from build123d import *

# Parameters (mm, degrees)
F0_W      = 130.6354291737
F0_H      = 70.8588063717
F1_DEPTH  = 25.4
F2_W      = 21.0115239024
F2_H      = 16.2068661302
F3_DEPTH  = 139.7
F4_W      = 130.6354291737
F4_H      = 35.4294031858
F5_DEPTH  = 27.94
F7_DEPTH  = 157.48
F8_W      = 13.1810824387
F8_H      = 8.3256293517
F8_W_2    = 15.867670998
F9_DEPTH  = 147.32
F10_W     = 5.3731799126
F10_H     = 22.795913741
F11_DEPTH = 15.24
F13_DEPTH = 25.4
F14_W     = 5.5410936475
F14_H     = 23.0333786458
F15_DEPTH = 15.24
F17_DEPTH = 25.4
F19_DEPTH = 45.72


with BuildPart() as f1:
    # F0 (on Top) → F1 (new body)
    with BuildSketch(Plane.XY):
        with Locations((6.5485667437, -7.4720792472)):
            Rectangle(F0_W, F0_H)
    extrude(amount=F1_DEPTH)

    # F2 (on face) → F3 (cut)
    with BuildSketch(Plane.YZ.offset(71.8662813306)):
        with Locations((17.4515619874, 8.1034330651)):
            Rectangle(F2_W, F2_H)
    extrude(amount=-F3_DEPTH, mode=Mode.SUBTRACT)

    # F4 (on face) → F5 (join)
    with BuildSketch(Plane.XY.offset(25.4)):
        with Locations((6.5485667437, 10.2426223457)):
            Rectangle(F4_W, F4_H)
    extrude(amount=F5_DEPTH)

    # F6 (on face) → F7 (cut)
    with BuildSketch(Plane.YZ.offset(71.8662813306)):
        Polygon((12.0896529406, 53.34), (5.7090031914, 53.34), (5.7090031914, 36.6887412965), (-1.8470302457, 36.6887412965), (-1.8470302457, 31.315561384), (22.164363414, 31.315561384), (22.164363414, 36.6887412965), (12.0896529406, 36.6887412965), align=None)
    extrude(amount=-F7_DEPTH, mode=Mode.SUBTRACT)

    # F8 (on face) → F9 (cut)
    with BuildSketch(Plane.YZ.offset(71.8662813306)):
        with Locations((-0.8815380279, 49.1771853241)):
            Rectangle(F8_W, F8_H)
        with Locations((20.0234884396, 49.1771853241)):
            Rectangle(F8_W_2, F8_H)
    extrude(amount=-F9_DEPTH, mode=Mode.SUBTRACT)

    # F10 (on face) → F11 (join)
    with BuildSketch(Plane.XY.offset(25.4)):
        with Locations((-44.3287305534, -18.8700361177)):
            Rectangle(F10_W, F10_H)
    extrude(amount=F11_DEPTH)

    # F12 (on face) → F13 (cut)
    with BuildSketch(Plane(origin=(-47.0153205097, 0, 0), x_dir=(0, -1, 0), z_dir=(-1, 0, 0))):
        Polygon((30.2679929882, 40.64), (7.4720792472, 40.64), (30.2679929882, 25.4), align=None)
    extrude(amount=-F13_DEPTH, mode=Mode.SUBTRACT)

    # F14 (on face) → F15 (join)
    with BuildSketch(Plane.XY.offset(25.4)):
        with Locations((60.7001371682, -18.9887685701)):
            Rectangle(F14_W, F14_H)
    extrude(amount=F15_DEPTH)

    # F16 (on face) → F17 (cut)
    with BuildSketch(Plane(origin=(57.9295903444, 0, 0), x_dir=(0, -1, 0), z_dir=(-1, 0, 0))):
        Polygon((30.505457893, 40.64), (7.4720792472, 40.64), (30.505457893, 25.4), align=None)
    extrude(amount=-F17_DEPTH, mode=Mode.SUBTRACT)

    # F18 (on face) → F19 (cut)
    with BuildSketch(Plane.XY.offset(25.4)):
        with BuildLine():
            Line((-5.2471338319, -21.9567809254), (2.8545020614, -21.9567809254))
            Line((2.8545020614, -21.9567809254), (2.8545020614, -13.8551450321))
            ThreePointArc((2.8545020614, -13.8551450321), (-2.8742196175, -16.2280592466), (-5.2471338319, -21.9567809254))
        make_face()
        with BuildLine():
            Line((2.8545020614, -13.8551450321), (2.8545020614, -21.9567809254))
            Line((2.8545020614, -21.9567809254), (10.9561379547, -21.9567809254))
            ThreePointArc((10.9561379547, -21.9567809254), (8.5832237402, -16.2280592466), (2.8545020614, -13.8551450321))
        make_face()
        with BuildLine():
            Line((2.8545020614, -30.0584168187), (2.8545020614, -21.9567809254))
            Line((2.8545020614, -21.9567809254), (-5.2471338319, -21.9567809254))
            ThreePointArc((-5.2471338319, -21.9567809254), (-2.8742196175, -27.6855026042), (2.8545020614, -30.0584168187))
        make_face()
        with BuildLine():
            Line((10.9561379547, -21.9567809254), (2.8545020614, -21.9567809254))
            Line((2.8545020614, -21.9567809254), (2.8545020614, -30.0584168187))
            ThreePointArc((2.8545020614, -30.0584168187), (8.5832237402, -27.6855026042), (10.9561379547, -21.9567809254))
        make_face()
    extrude(amount=-F19_DEPTH, mode=Mode.SUBTRACT)


solid = f1.part
Source: CAD feature listing. Evaluate the final solid. Frame: model axes, mm. A direction names the side the tool comes from. Coordinates: 2 decimals unless noted, no trailing zeros. Loops run counter-clockwise (first coordinate to the right, second up) from the corner with the lowest first, then second, coordinate; pieces in that order, holes last. Notation, with made-up numbers: M 62.5,29 L 100.5,29 A18 ccw 100.5,46 Z; hole C -37.75,46 d7. An arc over 180 degrees is marked long. Answer in a Markdown table with one row per item.
Q1. Draft query along Z for faces 5 (the flat face through (7, 2, 36.689)), 6 (the flat face through (7, 12.09, 41)), 7 (the flat face through (7, -1, 45.014)), 8 (the flat face through (6, -12, 0)). Return one class per face: pulls with the +Z half, pulls with the -Z half, needs draft (parallel to the pull), parting line crosses it, or undercut.
Answers below:
| item | result |
|---|---|
| face 5 | undercut |
| face 6 | needs draft |
| face 7 | pulls with the +Z half |
| face 8 | pulls with the -Z half |
Q2. Section D-D on x = 22. Return the cut outline in (y, z), plus the area to 3 significant figures.
Answers below:
| item | result |
|---|---|
| outline | M -42.9,0 L 6.95,0 L 6.95,16.21 L 27.96,16.21 L 27.96,45.01 L 12.09,45.01 L 12.09,36.69 L 22.16,36.69 L 22.16,31.32 L -1.85,31.32 L -1.85,36.69 L 5.71,36.69 L 5.71,45.01 L -7.47,45.01 L -7.47,25.4 L -42.9,25.4 Z |
| area | 1,970 mm^2 |
Q3. First-contact query: pin 1 (4.5 mm diameter, centred on x = 36, z = 34, fed in from -Y); pin 2 (4.5 mm diameter, centred on y = -17.5, z = 36.5, fed in from -X); pin 3 (3 mm diameter, centred on x = 45, y = -11.5, fed in from +Z). Flat tips, straight axial feed; report the tip coordinate or a pass-through.
Answers below:
| item | result |
|---|---|
| pin 1 | stops at y = -7.47 |
| pin 2 | stops at x = -47.02 |
| pin 3 | stops at z = 25.4 |
Q4. Set-up query: faces 1 (the flat face through (63.471, -14, 30)), 2 (the flat face through (7, 17, 36.689)), 3 (the flat face through (7, 17, 16.207)), 4 (the flat face through (-41.642, -14, 30)). Return all of +Z, -Z, +X, -X, +Y, -Y with unobstructed straight access to the full face (end or side cutting, diameter ignored); none if empty.
Answers below:
| item | result |
|---|---|
| face 1 | +Z, +X, -Y |
| face 2 | +X, -X |
| face 3 | -Z, +X, -X, +Y |
| face 4 | +Z, -Y |
Q5. Section B-B on z = 8. Return the cut outline in (x, y).
Answers below:
| item | result |
|---|---|
| outline | M -58.77,-42.9 L 71.87,-42.9 L 71.87,6.95 L -58.77,6.95 Z; hole C 2.85,-21.96 d16.2 |
Q6. Section C-C on z = 42. Return the cut outline in (x, y), plus the area to 3 significant figures.
Answers below:
| item | result |
|---|---|
| outline | M -58.77,-7.47 L 71.87,-7.47 L 71.87,5.71 L -58.77,5.71 Z; M -58.77,12.09 L 71.87,12.09 L 71.87,27.96 L -58.77,27.96 Z |
| area | 3,790 mm^2 |
Q7. Section A-A on y = 14. Return the cut outline in (x, z).
Answers below:
| item | result |
|---|---|
| outline | M -58.77,16.21 L 71.87,16.21 L 71.87,31.32 L -58.77,31.32 Z; M -58.77,36.69 L 71.87,36.69 L 71.87,45.01 L -58.77,45.01 Z |
Q8. Ray query, probe 1 along Z at (x, y) = (12, 0.5); probe 2 along Z at (x, y) = (58.5, 14); probe 3 along Z at (x, y) = (23, 8.5). Return the intervals inside material, ascending. Write a range as from..to.
Answers below:
| item | result |
|---|---|
| probe 1 | z = 0..31.32, 36.69..45.01 |
| probe 2 | z = 16.21..31.32, 36.69..45.01 |
| probe 3 | z = 16.21..31.32 |
